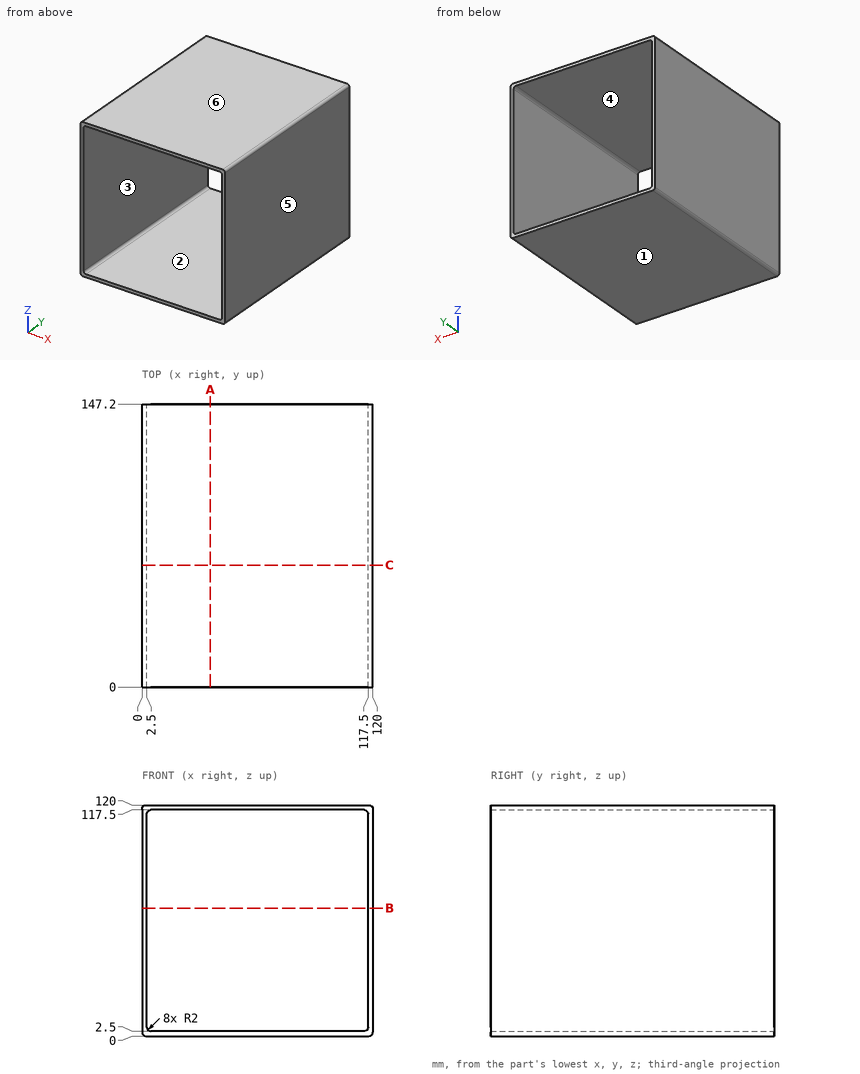
Could you check a few things on this drawing? It's one solid part, dimensions in mm from its lowest x, y, z. A direction names the side the tool comes from. Coordinates: 2 decimals unless noted, no trailing zeros. Write each loop counter-clockwise with the first axis right and the second up, starting at its lowest first coordinate (ties: lowest second). Pieces come first, ordered by that corner, then holes. Notation, with made-up numbers: (-4, 30) - (22, 30) arc R17 ccw to (22, 37) - close; hole circle Ø4 at (-38, 88.5). An arc over 180 degrees is marked (long way). Return JSON: item names as keys, results as strings. Group by question number.
Item 1: If we section it at B-B (z = 66.5): Write out the boundary of the cut face in (x, y).
Item 2: We'd pull the mould along X, two halves only. Please class the marked faces 3, 4, 5 and 6: pulls with the +X half, pulls with the -X half, needs draft (parallel to the pull), parting line crosses it, or undercut.
Item 3: If we section it at C-C (y = 63.5): Write out the boundary of the cut face in (x, z), then the cut area to 4 significant figures.
Item 4: If we section it at A-A (x = 35.5): Write out the boundary of the cut face in (y, z).
Item 5: I'm going to push a flat-ended pin straight in: pin 1 Ø6 at (x, y) = (51, 27.5) entering from -Z. Where does the tip first touch, or does it pass through?
Item 6: Please list where this line runs through material, in increasing order: probe 1 along Z at (x, y) = (107.5, 89.5).
Item 7: Which directions (+Z, -Z, +X, -X, +Y, -Y) give clear straight access to the entire face, cutting with the end or side of a thin tool? Please do the marked faces 1 and 2.
Return value:
{
 "1": {"outline": "(0, 0) - (2.5, 0) - (2.5, 147.2) - (0, 147.2) - close; (117.5, 0) - (120, 0) - (120, 147.2) - (117.5, 147.2) - close"},
 "2": {"face 3": "undercut", "face 4": "undercut", "face 5": "pulls with the +X half", "face 6": "needs draft"},
 "3": {"outline": "(0, 2) arc R2 ccw to (2, 0) - (118, 0) arc R2 ccw to (120, 2) - (120, 118) arc R2 ccw to (118, 120) - (2, 120) arc R2 ccw to (0, 118) - close; hole (2.5, 4.5) arc R2 ccw to (4.5, 2.5) - (115.5, 2.5) arc R2 ccw to (117.5, 4.5) - (117.5, 115.5) arc R2 ccw to (115.5, 117.5) - (4.5, 117.5) arc R2 ccw to (2.5, 115.5) - close", "area": "1,175 mm^2"},
 "4": {"outline": "(0, 0) - (147.2, 0) - (147.2, 2.5) - (0, 2.5) - close; (0, 117.5) - (147.2, 117.5) - (147.2, 120) - (0, 120) - close"},
 "5": {"pin 1": "stops at z = 0"},
 "6": {"probe 1": "z = 0 to 2.5, 117.5 to 120"},
 "7": {"face 1": "-Z, +X, -X, +Y, -Y", "face 2": "+Y, -Y"}
}
